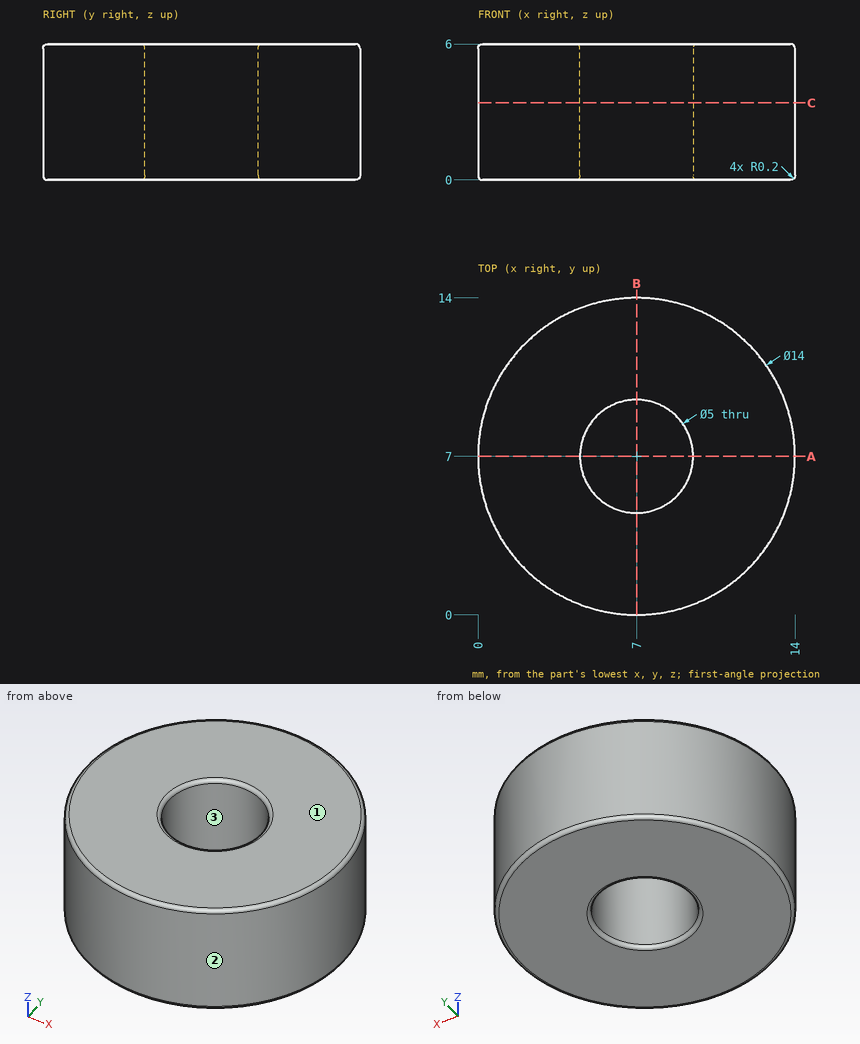
Geometry check sheet. Reference: drawing and pictorial views, mm from the part's lowest x, y, z. Round coordinates to 2 decimals unless told otherwise and drop trailing zeros. Loops run counter-clockwise (first coordinate to the right, second up) from the corner with the lowest first, then second, coordinate; pieces in that order, holes last.
1. Sectioned sample at C-C on z = 3.4. Record the boundary of the cut face in (x, y), and give its area (3 significant figures).
2. Scan lines: probe 1 along Y at (x, z) = (7, 2.75); probe 2 along Y at (x, z) = (9, 4.3); probe 3 along X at (y, z) = (6.25, 0.95). Record each from-to range of solid material in increasing order.
3. Mould release check, pull along X, two halves, no side actions. Record for the marked faces 1, 2 and 3: released by +X, released by -X, zero draft, split by the parting line, or undercut.
4. Sectioned sample at A-A on y = 7. Record the boundary of the cut face in (x, z).
Recorded:
1. outline: circle Ø14 at (7, 7); hole circle Ø5 at (7, 7)
1. area: 134 mm2
2. probe 1: y = 0 to 4.5, 9.5 to 14
2. probe 2: y = 0.29 to 5.5, 8.5 to 13.71
2. probe 3: x = 0.04 to 4.62, 9.38 to 13.96
3. face 1: zero draft
3. face 2: split by the parting line
3. face 3: undercut
4. outline: (0, 0.2) arc R0.2 ccw to (0.2, 0) - (4.3, 0) arc R0.2 ccw to (4.5, 0.2) - (4.5, 5.8) arc R0.2 ccw to (4.3, 6) - (0.2, 6) arc R0.2 ccw to (0, 5.8) - close; (9.5, 0.2) arc R0.2 ccw to (9.7, 0) - (13.8, 0) arc R0.2 ccw to (14, 0.2) - (14, 5.8) arc R0.2 ccw to (13.8, 6) - (9.7, 6) arc R0.2 ccw to (9.5, 5.8) - close
